Here's how the part is built. I have some questions about the finished solid (model axes, mm). Face numbers are marked on the shaded views. A direction names the side the tool comes from. Round coordinates to 2 decimals unless told otherwise and drop trailing zeros. Order: outer loops, then holes, each group sorted by start corner. A loop starts at its lowest first (then second) coordinate and runs counter-clockwise, first axis right, second up. Notation, with made-up numbers: (9, 57) -> (47, 57) arc R11 ccw to (47, 66) -> close; hole circle Ø7 at (25.25, 89.25). An arc over 180 degrees is marked (long way). Answer in a Markdown table with one row per item.
Autodesk Inventor part; units mm, degrees
ref_plane "YZ Plane" through (0, 0, 0) normal (1, 0, 0) x (0, 1, 0)
ref_plane "XZ Plane" through (0, 0, 0) normal (0, 1, 0) x (-1, 0, 0)
ref_plane "XY Plane" through (0, 0, 0) normal (0, 0, 1) x (1, 0, 0)
sketch "Sketch1" plane through (0, 0, 0) normal (1, 0, 0) x (0, 1, 0)
  line L0 (-78.9055, 475.022) -> (-258.9055, 475.022)
  line L1 (-258.9055, 475.022) -> (-258.9055, 439.022)
  line L2 (-258.9055, 439.022) -> (-78.9055, 439.022)
  line L3 (-78.9055, 439.022) -> (-78.9055, 475.022)
  point P0 (0, 0)
  dimension "d0" = 180
  dimension "d1" = 36
extrude "Plate1" add sketch "Sketch1" along normal blind 0.5
sketch "Sketch2" plane through (0.5, -79.4055, 475.022) normal (0, 1, 0) x (1, 0, 0)
  line L0 (0, -36) -> (0, 0)
  line L1 (0, 0) -> (-36, 0)
  line L2 (-36, 0) -> (-36, -36)
  line L3 (-36, -36) -> (0, -36)
edge flange "Flange1" height 36 angle 90 thickness 0.5 bend radius 0.5 thickness toward (0, 1, 0) relief tear relief width 0.5 relief depth 0.25 edges at (0.5, -78.9055, 457.022) wall of the first edge with corners at (0.5, -79.4055, 439.022) (0.5, -79.4055, 475.022) (-35.5, -79.4055, 475.022) (-35.5, -79.4055, 439.022)
bend "Bend1"
corner "Corner1"
sketch "Sketch3" plane through (-35, -78.9055, 475.022) normal (-1, 0, 0) x (0, 1, 0)
  line L0 (0, -36) -> (0, 0)
  line L1 (0, 0) -> (-180, 0)
  line L2 (-180, 0) -> (-180, -36)
  line L3 (-180, -36) -> (0, -36)
edge flange "Flange2" height 180 angle 90 thickness 0.5 bend radius 0.5 thickness toward (-1, 0, 0) relief tear relief width 0.5 relief depth 0.25 edges at (-35.5, -78.9055, 457.022) wall of the first edge with corners at (-35, -78.9055, 439.022) (-35, -78.9055, 475.022) (-35, -258.9055, 475.022) (-35, -258.9055, 439.022)
bend "Bend2"
corner "Corner2"
sketch "Sketch4" plane through (-35, -258.4055, 439.022) normal (0, -1, 0) x (-1, 0, 0)
  line L0 (0, 36) -> (0, 0)
  line L1 (0, 0) -> (25, 0)
  line L2 (25, 0) -> (25, 36)
  line L3 (25, 36) -> (0, 36)
edge flange "Flange3" height 25 angle 90 thickness 0.5 bend radius 0.5 thickness toward (0, -1, 0) relief tear relief width 0.5 relief depth 0.25 edges at (-35, -258.9055, 457.022) wall of the first edge with corners at (-35, -258.4055, 475.022) (-35, -258.4055, 439.022) (-60, -258.4055, 439.022) (-60, -258.4055, 475.022)
bend "Bend3"
corner "Corner3"
sketch "Sketch5" plane through (-59.5, -258.9055, 475.022) normal (-1, 0, 0) x (0, -1, 0)
  line L0 (0, -36) -> (0, 0)
  line L1 (0, 0) -> (-80, 0)
  line L2 (-80, 0) -> (-80, -36)
  line L3 (-80, -36) -> (0, -36)
edge flange "Flange4" height 80 angle 90 thickness 0.5 bend radius 0.5 thickness toward (-1, 0, 0) relief tear relief width 0.5 relief depth 0.25 edges at (-60, -258.4055, 457.022) wall of the first edge with corners at (-59.5, -258.9055, 439.022) (-59.5, -258.9055, 475.022) (-59.5, -178.9055, 475.022) (-59.5, -178.9055, 439.022)
bend "Bend4"
corner "Corner4"
sketch "Sketch6" plane through (-59.5, -178.9055, 475.022) normal (1, 0, 0) x (0, 0, -1)
  point P0 (475.022, 178.9055)
  point P1 (18.2971, -1.4985)
hole "Hole1" at (-59.5, -180.404, 456.7249) direction (-1, 0, 0) diameter 33 depth 33 tip angle 118
sketch "Sketch7" plane through (-35, -79.9055, 475.022) normal (1, 0, 0) x (0, 0, -1)
  point P0 (475.022, 79.9055)
  point P1 (20.1704, -99.7704)
hole "Hole2" at (-35, -179.6759, 454.8516) direction (-1, 0, 0) diameter 12.2 depth 0.5 tip angle 118
sketch "Sketch8" plane through (-0.5, -78.9055, 475.022) normal (0, 1, 0) x (1, 0, 0)
  point P0 (0.5, 475.022)
  point P1 (-28.4213, 17.8782)
hole "Hole3" at (-28.9213, -78.9055, 457.1438) direction (0, -1, 0) diameter 6 depth 0.75 tip angle 118
sketch "Sketch9" plane through (-35.5, -79.9055, 439.022) normal (-1, 0, 0) x (0, 0, 1)
  point P0 (-439.022, 79.9055)
  point P1 (19.2457, -16.2545)
hole "Hole4" at (-35.5, -96.16, 458.2677) direction (1, 0, 0) diameter 6 depth 0.5 tip angle 118
equation "\"d55\" = Thickness"
equation "\"d69\" = Thickness"
equation "\"d2\" = Thickness"
equation "\"d3\" = BendReliefWidth"
equation "\"d4\" = BendReliefDepth"
equation "\"d5\" = MinimumRemnant"
equation "\"d6\" = TransitionRadius"
equation "\"d9\" = BendRadius"
equation "\"d10\" = CornerReliefSize"
equation "\"d11\" = GapSize"
equation "\"d12\" = JacobiRadiusSize"
equation "\"d13\" = BendReliefWidth"
equation "\"d14\" = BendReliefDepth"
equation "\"d15\" = MinimumRemnant"
equation "\"d16\" = TransitionRadius"
equation "\"d19\" = BendRadius"
equation "\"d20\" = CornerReliefSize"
equation "\"d21\" = GapSize"
equation "\"d22\" = JacobiRadiusSize"
equation "\"d23\" = BendReliefWidth"
equation "\"d24\" = BendReliefDepth"
equation "\"d25\" = MinimumRemnant"
equation "\"d26\" = TransitionRadius"
equation "\"d29\" = BendRadius"
equation "\"d30\" = CornerReliefSize"
equation "\"d31\" = GapSize"
equation "\"d32\" = JacobiRadiusSize"
equation "\"d33\" = BendReliefWidth"
equation "\"d34\" = BendReliefDepth"
equation "\"d35\" = MinimumRemnant"
equation "\"d36\" = TransitionRadius"
equation "\"d39\" = BendRadius"
equation "\"d40\" = CornerReliefSize"
equation "\"d41\" = GapSize"
equation "\"d42\" = JacobiRadiusSize"
equation "\"BendRadius\" = Thickness"
equation "\"BendReliefWidth\" = Thickness"
equation "\"BendReliefDepth\" = 0.5 * Thickness"
equation "\"CornerReliefSize\" = 4 * Thickness"
equation "\"MinimumRemnant\" = 2 * Thickness"
equation "\"TransitionRadius\" = BendRadius"
equation "\"JacobiRadiusSize\" = BendRadius"
equation "\"GapSize\" = Thickness"
properties part number "strikkkk"
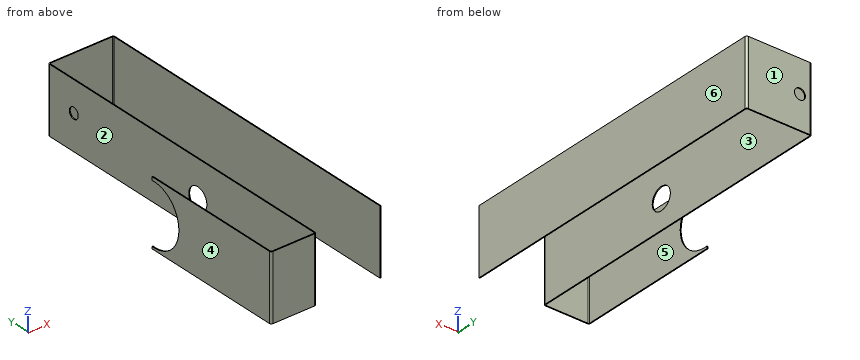
1. Please list where these lines run through material, in increasing order: line 1 along X through (y, z) = (-251, 461); line 2 along X through (y, z) = (-145, 443); line 3 along Y through (x, z) = (-58, 458).
Numbers:
| item | result |
|---|---|
| line 1 | x = -60 to -59.5, -35.5 to -35, 0 to 0.5 |
| line 2 | x = -35.5 to -35, 0 to 0.5 |
| line 3 | y = -258.91 to -258.41 |
2. Suppose I cut it at B-B on z = 457. State how many separate pieces and enclosed holes the cut face has, then the cut area to 3 significant figures.
Numbers:
| item | result |
|---|---|
| separate pieces | 4 |
| enclosed holes | 0 |
| area | 228 mm2 |
3. We'd pull the mould along X, two halves only. Please class the marked faces 4, 5 and 6: released by +X, released by -X, zero draft, split by the parting line, or undercut.
Numbers:
| item | result |
|---|---|
| face 4 | released by -X |
| face 5 | undercut |
| face 6 | released by +X |
4. Suppose I cut it at C-C on x = -48. Write out the boundary of the cut face in (y, z).
Numbers:
| item | result |
|---|---|
| outline | (-258.91, 439.02) -> (-258.41, 439.02) -> (-258.41, 475.02) -> (-258.91, 475.02) -> close |
5. Suppose I cut it at D-D on y = -204. Write out the boundary of the cut face in (x, z), then the cut area to 3 significant figures.
Numbers:
| item | result |
|---|---|
| outline | (-60, 439.02) -> (-59.5, 439.02) -> (-59.5, 475.02) -> (-60, 475.02) -> close; (-35.5, 439.02) -> (-35, 439.02) -> (-35, 475.02) -> (-35.5, 475.02) -> close; (0, 439.02) -> (0.5, 439.02) -> (0.5, 475.02) -> (0, 475.02) -> close |
| area | 54.0 mm2 |
6. For the marked faces 1, 2 and 3, which set-ups out of +Z, -Z, +X, -X, +Y, -Y let a thin tool reach every point of the face, with its end or its side?
Numbers:
| item | result |
|---|---|
| face 1 | +Z, -Z, +X, -X, +Y |
| face 2 | +Z, -Z, +Y |
| face 3 | +Z, -Z, -Y |
7. Suppose I cut it at A-A on y = -96.16. Write out the boundary of the cut face in (x, z).
Numbers:
| item | result |
|---|---|
| outline | (-35.5, 439.02) -> (-35, 439.02) -> (-35, 455.27) -> (-35.5, 455.27) -> close; (-35.5, 461.27) -> (-35, 461.27) -> (-35, 475.02) -> (-35.5, 475.02) -> close; (0, 439.02) -> (0.5, 439.02) -> (0.5, 475.02) -> (0, 475.02) -> close |
8. For pin 1 Ø0.6 at (x, z) = (-60, 439.5) entering from +Y; pin 2 Ø4 at (x, y) = (-36.5, -200) entering from -Z; pin 3 Ø5.5 at (y, z) = (-96.16, 458.27) entering from -X; pin 4 Ø4 at (x, z) = (-20, 465.5) entering from -Y, each with a flat end and sliding along its axis, tell me the tip position at first contact or that it passes through.
Numbers:
| item | result |
|---|---|
| pin 1 | stops at y = -178.91 |
| pin 2 | stops at z = 439.02 |
| pin 3 | stops at x = 0 |
| pin 4 | stops at y = -79.41 |
